```python
from build123d import *

# Parameters (mm, degrees)
SKETCH1_W           = 105
SKETCH1_H           = 80
BOSS_EXTRUDE1_DEPTH = 3
SKETCH3_R           = 3.75
CUT_EXTRUDE1_DEPTH  = 2.2
SKETCH4_W           = 10
SKETCH4_H           = 4
SKETCH4_W_2         = 4
SKETCH4_H_2         = 10
CUT_EXTRUDE2_DEPTH  = 10
FILLET2_R           = 3
FILLET3_R           = 3


with BuildPart() as part:
    # Sketch1 → Boss-Extrude1 (new body)
    with BuildSketch(Plane.XY):
        Rectangle(SKETCH1_W, SKETCH1_H)
    extrude(amount=BOSS_EXTRUDE1_DEPTH)

    # Sketch3 → Cut-Extrude1 (cut)
    with BuildSketch(Plane(origin=(0, 0, 0), x_dir=(-1, 0, 0), z_dir=(0, 0, -1))):
        with Locations((-24.509514806, 24.509514806)):
            Circle(SKETCH3_R)
        with Locations((24.509514806, 24.509514806)):
            Circle(SKETCH3_R)
        with Locations((24.509514806, -24.509514806)):
            Circle(SKETCH3_R)
        with Locations((-24.509514806, -24.509514806)):
            Circle(SKETCH3_R)
    extrude(amount=-CUT_EXTRUDE1_DEPTH, mode=Mode.SUBTRACT)

    # Sketch4 → Cut-Extrude2 (cut)
    with BuildSketch(Plane.XY.offset(3)):
        with Locations((-0.446296315, 35.38913846)):
            Rectangle(SKETCH4_W, SKETCH4_H)
        with Locations((-0.446296315, -35.324542102)):
            Rectangle(SKETCH4_W, SKETCH4_H)
        with Locations((-35.586810408, 0.617671805)):
            Rectangle(SKETCH4_W_2, SKETCH4_H_2)
        with Locations((34.669298403, 0.617671805)):
            Rectangle(SKETCH4_W_2, SKETCH4_H_2)
    extrude(amount=-CUT_EXTRUDE2_DEPTH, mode=Mode.SUBTRACT)

    # Fillet2
    fillet2_edges = [part.edges().sort_by_distance(p)[0] for p in [
        (-52.5, -40, 1.5),
    ]]
    fillet(fillet2_edges, radius=FILLET2_R)

    # Fillet3
    fillet3_edges = [part.edges().sort_by_distance(p)[0] for p in [
        (-52.5, 40, 1.5),
        (52.5, 40, 1.5),
        (52.5, -40, 1.5),
    ]]
    fillet(fillet3_edges, radius=FILLET3_R)


solid = part.part
```
Work out the finished part from the listing and answer in its coordinate system (mm). A direction names the side the tool comes from. Coordinates: 2 decimals unless noted, no trailing zeros. Order: outer loops, then holes, each group sorted by start corner. A loop starts at its lowest first (then second) coordinate and runs counter-clockwise, first axis right, second up. Notation, with made-up numbers: M 42.25,68.5 L 77.25,68.5 A26 cw 77.25,92.5 Z; hole C 29,11 d6. An arc over 180 degrees is marked long. Use CSV: the item, a comma, the result in double quotes.
1) Section B-B on z = 0.85 is taken. Count the separate pieces of the cut face and the enclosed holes in it, plus the area to 3 significant figures.
Worked out:
separate pieces,"1"
enclosed holes,"8"
area,"8,060 mm^2"
2) A flat-ended cylindrical pin translates along its axis: pin 1 Ø4 at (x, y) = (-25.5, -23.5) entering from -Z. Find the tip coordinate at first contact, or state that the pin passes through.
Worked out:
pin 1,"stops at z = 2.2"
3) Section C-C on y = -22.5 is taken. Write down the section's boundary in (x, z).
Worked out:
outline,"M -52.5,0 L -27.68,0 L -27.68,2.2 L -21.34,2.2 L -21.34,0 L 21.34,0 L 21.34,2.2 L 27.68,2.2 L 27.68,0 L 52.5,0 L 52.5,3 L -52.5,3 Z"
4) Section A-A on x = -3.5 is taken. Write down the section's boundary in (y, z).
Worked out:
outline,"M -40,0 L -37.32,0 L -37.32,3 L -40,3 Z; M -33.32,0 L 33.39,0 L 33.39,3 L -33.32,3 Z; M 37.39,0 L 40,0 L 40,3 L 37.39,3 Z"
5) Consider line 1 (Y direction, x = -0.5, z = 1.1); line 2 (X direction, y = 0.5, z = 1.05); line 3 (Y direction, x = -37, z = 2.4). Determine where each line is inside the solid, lowest interval first. Write a range as [from, to].
Worked out:
line 1,"y = [-40, -37.32], [-33.32, 33.39], [37.39, 40]"
line 2,"x = [-52.5, -37.59], [-33.59, 32.67], [36.67, 52.5]"
line 3,"y = [-40, -4.38], [5.62, 40]"
6) For faces 4 (the face through (-24, -24, 2.2)), 5 (the face through (-51.64, 39.1, 1.52)), 6 (the face through (32.669, 1, 2)), determine the directions among +Z, -Z, +X, -X, +Y, -Y from which every point of the face is accessible in a straight line to the end or side of a thin tool.
Worked out:
face 4,"-Z"
face 5,"+Z, -Z, -X, +Y"
face 6,"+Z, -Z"
7) Determine the mould class of faces 1 (the face through (28.256, -24.345, 1.085)), 2 (the face through (51.6, -39.14, 1.52)), 3 (the face through (-1, 1, 3)) for opening direction Y: released by +Y, released by -Y, zero draft, split by the parting line, or undercut.
Worked out:
face 1,"undercut"
face 2,"released by -Y"
face 3,"zero draft"
